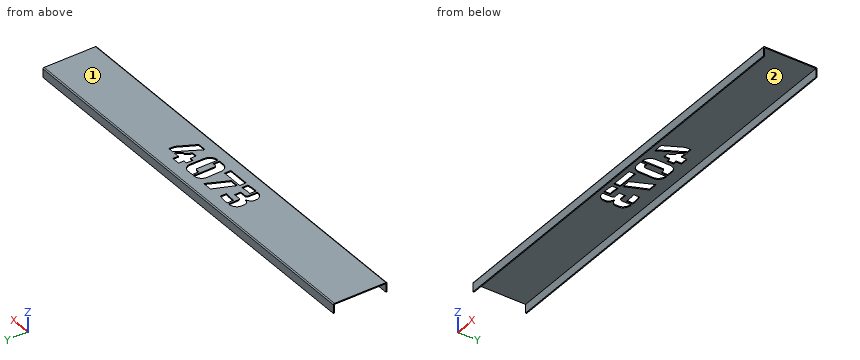
Autodesk Inventor part; units mm, degrees
ref_plane "YZ Plane" through (0, 0, 0) normal (1, 0, 0) x (0, 1, 0)
ref_plane "XZ Plane" through (0, 0, 0) normal (0, 1, 0) x (-1, 0, 0)
ref_plane "XY Plane" through (0, 0, 0) normal (0, 0, 1) x (1, 0, 0)
sketch "Sketch1" plane through (0, 0, 0) normal (0, 0, 1) x (1, 0, 0)
  line L0 (0, 0) -> (609.6, 0)
  line L1 (609.6, 0) -> (609.6, 76.2)
  line L2 (609.6, 76.2) -> (0, 76.2)
  line L3 (0, 76.2) -> (0, 0)
  dimension "d0" = 609.6
  dimension "d1" = 76.2
extrude "Extrusion1" add sketch "Sketch1" along normal blind 1.5875
sketch "Sketch2" plane through (0, 76.2, 0) normal (0, 1, 0) x (1, 0, 0)
  line L0 (609.6, 0) -> (0, 0)
  line L1 (0, 0) -> (0, -1.5875)
  line L2 (609.6, -1.5875) -> (0, -1.5875)
  line L3 (609.6, 0) -> (609.6, -1.5875)
  line L4 (609.6, -1.5875) -> (0, -1.5875)
  line L5 (0, -1.5875) -> (0, 12.7)
  line L6 (0, 12.7) -> (609.6, 12.7)
  line L7 (609.6, 12.7) -> (609.6, -1.5875)
  dimension "d39" = 12.7
extrude "Extrusion2" add sketch "Sketch2" along normal blind 1.5875
fillet "Fillet1" radius 1.5875 1 edges at (304.8, 77.7875, 1.5875)
sketch "Sketch3" plane through (0, 0, 0) normal (0, -1, 0) x (1, 0, 0)
  line L0 (609.6, 0) -> (0, 0)
  line L1 (0, -12.7) -> (0, 0)
  line L2 (609.6, -12.7) -> (0, -12.7)
  line L3 (609.6, 0) -> (609.6, -12.7)
extrude "Extrusion3" add sketch "Sketch3" along normal blind 1.5875
sketch "Sketch4" plane through (0, 76.2, -12.7) normal (-1, 0, 0) x (0, 0, 1)
  line L0 (12.7, -76.2) -> (0, -76.2)
  line L1 (0, -76.2) -> (0, -77.7875)
  line L2 (12.7, -77.7875) -> (0, -77.7875)
  line L3 (12.7, -76.2) -> (12.7, -77.7875)
  arc A0 (14.2875, 0) -> (12.7, 1.5875) centre (12.7, 0) ccw
  line L4 (0, 1.5875) -> (12.7, 1.5875)
  line L5 (0, 0) -> (0, 1.5875)
  line L6 (0, 0) -> (12.7, 0)
  line L7 (12.7, 0) -> (12.7, -76.2)
  line L8 (12.7, -76.2) -> (14.2875, -76.2)
  line L9 (14.2875, -76.2) -> (14.2875, 0)
  line L10 (12.7, -76.2) -> (14.2875, -76.2)
  line L11 (14.2875, -76.2) -> (14.2875, -77.7875)
  line L12 (14.2875, -77.7875) -> (12.7, -77.7875)
  line L13 (12.7, -77.7875) -> (12.7, -76.2)
extrude "Extrusion4" add sketch "Sketch4" against normal up to surface (609.6 mm away) contours L8 L11 L12 L3
fillet "Fillet2" radius 1.5875 1 edges at (304.8, -1.5875, 1.5875)
sketch "Sketch5" plane through (0, 0, 1.5875) normal (0, 0, 1) x (1, 0, 0)
  line L0 (391.8077, 9.2075) -> (217.7923, 9.2075) construction
  line L1 (217.7923, 9.2075) -> (217.7923, 67.0009) construction
  line L2 (217.7923, 67.0009) -> (391.8077, 67.0009) construction
  line L3 (391.8077, 67.0009) -> (391.8077, 9.2075) construction
  line L4 (368.7246, 16.9668) -> (355.2902, 16.9668)
  line L5 (355.2902, 16.9668) -> (374.313, 51.6075)
  line L6 (366.0229, 42.0591) -> (362.766, 42.0591)
  line L7 (362.766, 42.0591) -> (358.2013, 33.4623)
  line L8 (358.2013, 33.4623) -> (350.738, 33.4623)
  line L9 (345.5567, 42.0591) -> (345.5567, 51.6075)
  line L10 (345.5567, 51.6075) -> (350.738, 51.6075)
  line L11 (350.738, 51.6075) -> (350.738, 59.6755)
  line L12 (350.738, 59.6755) -> (362.766, 59.6755)
  line L13 (362.766, 59.6755) -> (362.766, 51.6075)
  line L14 (362.766, 51.6075) -> (371.6483, 51.6075)
  line L15 (371.6483, 51.6075) -> (366.0229, 42.0591)
  line L16 (283.8325, 28.8388) -> (297.8915, 59.6755)
  line L17 (283.8325, 59.6755) -> (270.9618, 28.8388)
  line L18 (270.9618, 28.8388) -> (283.8325, 28.8388)
  line L19 (301.3907, 16.9668) -> (301.3907, 26.3815)
  line L20 (301.3907, 26.3815) -> (269.4747, 26.3815)
  line L21 (301.3907, 16.9668) -> (269.4747, 16.9668)
  line L22 (328.4185, 16.8456) -> (328.4185, 47.9611)
  line L23 (321.4042, 50.2314) -> (321.4042, 60.0732)
  line L24 (340.8479, 47.9611) -> (340.8479, 28.9034)
  arc A0 (328.4185, 47.9611) -> (326.7126, 50.2314) centre (326.1181, 48.0086) ccw
  arc A1 (328.4185, 16.8456) -> (340.8479, 28.9034) centre (328.8598, 28.8258) ccw
  line L25 (318.8829, 60.0719) -> (318.8829, 29.6859)
  line L26 (325.6836, 26.3815) -> (325.6836, 16.781)
  line L27 (325.6836, 16.781) -> (319.4882, 16.781)
  arc A2 (306.7329, 27.5963) -> (319.4882, 16.781) centre (318.2151, 28.2088) ccw
  line L28 (306.7329, 27.5963) -> (306.252, 48.615)
  arc A3 (318.8829, 60.0719) -> (306.252, 48.615) centre (317.5294, 48.873) ccw
  line L29 (321.4042, 60.0732) -> (328.4185, 60.0732)
  arc A4 (340.8479, 47.9611) -> (328.4185, 60.0732) centre (329.7877, 49.0447) ccw
  line L30 (609.6, 0) -> (609.6, 76.2)
  line L31 (0, 0) -> (0, 76.2)
  line L32 (609.6, 0) -> (0, 0)
  line L33 (0, 76.2) -> (609.6, 76.2)
  line L34 (297.8915, 59.6755) -> (283.8325, 59.6755)
  line L35 (269.4747, 26.3815) -> (269.4747, 16.9668)
  line L36 (326.7126, 50.2314) -> (321.4042, 50.2314)
  line L37 (368.7246, 16.9668) -> (382.3802, 43.1657)
  line L38 (382.3802, 43.1657) -> (382.5469, 51.6075)
  line L39 (382.5469, 51.6075) -> (374.313, 51.6075)
  line L40 (345.5567, 42.0591) -> (350.738, 42.0591)
  line L41 (350.738, 42.0591) -> (350.738, 33.4623)
  arc A5 (318.8829, 29.6859) -> (321.6099, 25.999) centre (321.7802, 28.9769) ccw
  arc A6 (321.6099, 25.999) -> (325.6836, 26.3815) centre (322.9641, 33.4611) ccw
  line L42 (257.2547, 33.4734) -> (257.2547, 42.6715)
  line L43 (257.2547, 42.6715) -> (247.6149, 42.6715)
  line L44 (245.5572, 46.0253) -> (245.5572, 59.7083)
  line L45 (233.0099, 52.0098) -> (233.0099, 45.4817)
  line L46 (240.4004, 38.1857) -> (240.4004, 37.57)
  line L47 (233.3728, 30.9594) -> (233.3728, 25.8822)
  line L48 (245.5572, 16.9419) -> (245.7765, 30.5952)
  arc A7 (233.3728, 25.8822) -> (245.5572, 16.9419) centre (245.0741, 29.0566) ccw
  arc A8 (240.4004, 37.57) -> (233.3728, 30.9594) centre (241.8707, 28.9661) ccw
  arc A9 (233.0099, 45.4817) -> (240.4004, 38.1857) centre (240.5679, 45.7465) ccw
  line L49 (257.2547, 33.4734) -> (248.2741, 33.4734)
  arc A10 (248.2741, 33.4734) -> (245.7765, 30.5952) centre (248.2741, 30.9507) ccw
  arc A11 (245.5572, 46.0253) -> (247.6149, 42.6715) centre (248.5719, 45.5669) ccw
  arc A12 (245.5572, 59.7083) -> (233.0099, 52.0098) centre (243.9929, 48.1836) ccw
  line L50 (264.4301, 17.9919) -> (264.4301, 26.8729)
  arc A13 (254.6467, 16.781) -> (264.4301, 17.9919) centre (253.1662, 68.8681) ccw
  line L51 (248.5719, 25.999) -> (248.5719, 16.781)
  line L52 (248.5719, 16.781) -> (254.6467, 16.781)
  arc A14 (248.5719, 25.999) -> (264.4301, 26.8729) centre (252.074, 106.7711) ccw
  arc A15 (264.6926, 49.5598) -> (248.2741, 50.5346) centre (251.6559, -31.2579) ccw
  line L53 (248.2741, 50.5346) -> (248.0544, 60.0732)
  line L54 (248.0544, 60.0732) -> (252.074, 60.1658)
  line L55 (264.6926, 49.5598) -> (264.6926, 58.3373)
  arc A16 (264.6926, 58.3373) -> (252.074, 60.1658) centre (243.9281, -40.5085) ccw
  point P0 (0, 38.1)
  point P1 (217.7923, 38.1042)
extrude "Extrusion9" cut sketch "Sketch5" against normal blind 25.4 contours L4 L5 L39 L38 L37 | L6 L7 L8 L41 L40 L9 L10 L11 L12 L13 L14 L15 | L18 L17 L34 L16 | L21 L35 L20 L19 | L22 A0 L36 L23 L29 A4 L24 A1 | L25 A5 A6 L26 L27 A2 L28 A3 | L49 A10 L48 A7 L47 A8 L46 A9 L45 A12 L44 A11 L43 L42 | A13 L52 L51 A14 L50 | A15 L53 L54 A16 L55
properties part number "Chassis FrontandBack"
Design review of the part built by this model. Coordinates are the model's own, in mm. Face numbers are marked on the shaded views. Round coordinates to 2 decimals unless told otherwise and drop trailing zeros. Write each loop counter-clockwise with the first axis right and the second up, starting at its lowest first coordinate (ties: lowest second). Pieces come first, ordered by that corner, then holes. Notation, with made-up numbers: (42, -10) -> (99, -10) arc R11 ccw to (99, -1) -> close; hole circle Ø3 at (69, 51). An arc over 180 degrees is marked (long way). Write item = value, one per line. Start each with the question number.
1) Mouldability with a two-part tool opening along Y and no side actions: class the marked faces 1 and 2 as +Y half, -Y half, draft (parallel to the pull), parting line (faces both ways), or undercut.
2) Take a section at B-B, the plane x = 553. State the section outline as (y, z) points (1 decimal).
3) Wall thickness on probe 1 along Y at (x, z) = (64, -7.75); probe 2 along Y at (x, z) = (367.5, 1); probe 3 along Z at (x, y) = (446, 3): over which ranges is each line inside the solid? List them lowest first. Write a range as from..to.
4) Clearance check with flat-ended pins moving along their axes: pin 1 (0.5 mm diameter, centred on x = 376.5, z = 0.5, fed in from -Y); pin 2 (0.5 mm diameter, centred on x = 254.5, z = 1, fed in from -Y); pin 3 (0.5 mm diameter, centred on x = 292.5, z = 1, fed in from +Y). State where each tip first meets the part, or that it passes through.
5) Take a section at A-A, the plane z = -7. State the section outline as (x, y) points, plus the area to 3 significant figures.
Results list:
q1.face_1 = draft
q1.face_2 = undercut
q2.outline = (-1.6, -12.7) -> (0, -12.7) -> (0, 0) -> (76.2, 0) -> (76.2, -12.7) -> (77.8, -12.7) -> (77.8, 0) arc R1.6 ccw to (76.2, 1.6) -> (0, 1.6) arc R1.6 ccw to (-1.6, 0) -> close
q3.probe_1 = -1.59..0, 76.2..77.79
q3.probe_2 = -1.23..16.97, 39.2..44.57, 51.61..77.43
q3.probe_3 = 0..1.59
q4.pin_1 = -1.57
q4.pin_2 = -1.4
q4.pin_3 = 77.6
q5.outline = (0, -1.59) -> (609.6, -1.59) -> (609.6, 0) -> (0, 0) -> close; (0, 76.2) -> (609.6, 76.2) -> (609.6, 77.79) -> (0, 77.79) -> close
q5.area = 1,940 mm²
